Autodesk Inventor part; units mm, degrees
ref_plane "YZ Plane" through (0, 0, 0) normal (1, 0, 0) x (0, 1, 0)
ref_plane "XZ Plane" through (0, 0, 0) normal (0, 1, 0) x (-1, 0, 0)
ref_plane "XY Plane" through (0, 0, 0) normal (0, 0, 1) x (1, 0, 0)
sketch "Skizze1" plane through (0, 0, 0) normal (0, 0, 1) x (1, 0, 0)
  line L0 (-80, 62.5) -> (80, 62.5)
  line L1 (80, 62.5) -> (80, -62.5)
  line L2 (80, -62.5) -> (-80, -62.5)
  line L3 (-80, -62.5) -> (-80, 62.5)
  line L4 (-80, 62.5) -> (80, -62.5) construction
  line L5 (80, 62.5) -> (-80, -62.5) construction
  point P0 (0, 0)
  dimension "d0" = 160
  dimension "d1" = 125
extrude "Extrusion1" add sketch "Skizze1" along normal blind 5
fillet "Rundung1" radius 20 4 edges at (80, 62.5, 2.5) (80, -62.5, 2.5) (-80, -62.5, 2.5) (-80, 62.5, 2.5)
sketch "Skizze2" plane through (0, 0, 5) normal (0, 0, 1) x (1, 0, 0)
  line L0 (6.6667, 14.6667) -> (14.6667, 14.6667)
  line L1 (14.6667, 14.6667) -> (14.6667, 6.6667)
  line L2 (14.6667, 6.6667) -> (6.6667, 6.6667)
  line L3 (6.6667, 6.6667) -> (6.6667, 14.6667)
  line L4 (6.6667, 14.6667) -> (14.6667, 6.6667) construction
  line L5 (14.6667, 14.6667) -> (6.6667, 6.6667) construction
  line L6 (2.6667, 18.6667) -> (18.6667, 18.6667)
  line L7 (18.6667, 18.6667) -> (18.6667, 2.6667)
  line L8 (18.6667, 2.6667) -> (2.6667, 2.6667)
  line L9 (2.6667, 2.6667) -> (2.6667, 18.6667)
  line L10 (2.6667, 18.6667) -> (18.6667, 2.6667) construction
  line L11 (18.6667, 18.6667) -> (2.6667, 2.6667) construction
  line L12 (-1.3333, 22.6667) -> (22.6667, 22.6667)
  line L13 (22.6667, 22.6667) -> (22.6667, -1.3333)
  line L14 (22.6667, -1.3333) -> (-1.3333, -1.3333)
  line L15 (-1.3333, -1.3333) -> (-1.3333, 22.6667)
  line L16 (-1.3333, 22.6667) -> (22.6667, -1.3333) construction
  line L17 (22.6667, 22.6667) -> (-1.3333, -1.3333) construction
  line L18 (-10.6667, -10.6667) -> (10.6667, -10.6667) construction
  line L19 (10.6667, -10.6667) -> (10.6667, 10.6667) construction
  line L20 (10.6667, 10.6667) -> (-10.6667, 10.6667) construction
  line L21 (-10.6667, 10.6667) -> (-10.6667, -10.6667) construction
  line L22 (-10.6667, -10.6667) -> (10.6667, 10.6667) construction
  line L23 (10.6667, -10.6667) -> (-10.6667, 10.6667) construction
  line L24 (60, 62.5) -> (-60, 62.5) construction
  line L25 (80, -42.5) -> (80, 42.5) construction
  line L26 (-14.6667, -14.6667) -> (-14.6667, -6.6667)
  line L27 (-14.6667, -6.6667) -> (-6.6667, -6.6667)
  line L28 (-6.6667, -6.6667) -> (-6.6667, -14.6667)
  line L29 (-6.6667, -14.6667) -> (-14.6667, -14.6667)
  line L30 (-6.6667, -6.6667) -> (-14.6667, -14.6667) construction
  line L31 (-2.6667, -2.6667) -> (-2.6667, -18.6667)
  line L32 (-18.6667, -2.6667) -> (-2.6667, -2.6667)
  line L33 (-18.6667, -18.6667) -> (-18.6667, -2.6667)
  line L34 (-2.6667, -18.6667) -> (-18.6667, -18.6667)
  line L35 (-2.6667, -2.6667) -> (-18.6667, -18.6667) construction
  line L36 (-18.6667, -2.6667) -> (-2.6667, -18.6667) construction
  line L37 (1.3333, -22.6667) -> (-22.6667, -22.6667)
  line L38 (-22.6667, 1.3333) -> (1.3333, 1.3333)
  line L39 (-22.6667, -22.6667) -> (-22.6667, 1.3333)
  line L40 (1.3333, 1.3333) -> (1.3333, -22.6667)
  line L41 (-22.6667, 1.3333) -> (1.3333, -22.6667) construction
  line L42 (1.3333, 1.3333) -> (-22.6667, -22.6667) construction
  line L43 (-14.6667, -6.6667) -> (-6.6667, -14.6667) construction
  point P0 (0, 0)
  point P1 (1.3333, -1.3333)
  point P2 (-1.3333, 1.3333)
  dimension "d14" = 8
  dimension "d15" = 8
  dimension "d16" = 16
  dimension "d17" = 16
  dimension "d18" = 24
  dimension "d20" = 21.3333
  dimension "d21" = 21.3333
  dimension "d22" = 62.5
  dimension "d23" = 80
  dimension "d24" = 8
  dimension "d25" = 8
  dimension "d26" = 16
  dimension "d27" = 16
  dimension "d28" = 24
extrude "Extrusion2" cut sketch "Skizze2" against normal blind 1.5
sketch "Skizze3" plane through (0, 0, 0) normal (0, 0, -1) x (-1, 0, 0)
  circle A0 centre (50, -53.5) radius 4
  line L0 (60, -62.5) -> (-60, -62.5)
  line L1 (80, 42.5) -> (80, -42.5)
  line L2 (50, -53.5) -> (-45.5, -53.5)
  line L3 (-45.5, -53.5) -> (-45.5, 25)
  line L4 (-45.5, 25) -> (50, 25)
  line L5 (50, 25) -> (50, -53.5)
  circle A1 centre (-45.5, -53.5) radius 4
  circle A2 centre (-45.5, 25) radius 4
  circle A3 centre (50, 25) radius 4
  circle A4 centre (-45.5, 25) radius 2
  circle A5 centre (50, 25) radius 2
  circle A6 centre (50, -53.5) radius 2
  circle A7 centre (-45.5, -53.5) radius 2
  point P0 (0, 0)
  dimension "d31" = 9
  dimension "d32" = 30
  dimension "d33" = 8
  dimension "d34" = 78.5
  dimension "d35" = 95.5
  dimension "d36" = 8
  dimension "d37" = 8
  dimension "d38" = 8
  dimension "d39" = 4
  dimension "d40" = 4
  dimension "d41" = 4
  dimension "d42" = 4
extrude "Extrusion3" add sketch "Skizze3" along normal blind 7 contours A0 L2 A6 L5 | L5 A6 L2 A0 | A3 L4 A5 L5 | L5 A5 L4 A3 | A1 L3 A7 L2 | L2 A7 L3 A1 | A2 L3 A4 L4 | L4 A4 L3 A2
sketch "Skizze4" plane through (0, 0, 0) normal (0, 0, -1) x (-1, 0, 0)
  line L0 (-80, -42.5) -> (-80, 42.5)
  line L1 (80, 42.5) -> (80, -42.5)
  line L2 (-77, 40) -> (-65, 40)
  line L3 (-65, 40) -> (-65, -40)
  line L4 (-65, -40) -> (-77, -40)
  line L5 (-77, -40) -> (-77, 40)
  line L6 (77, 40) -> (65, 40)
  line L7 (65, 40) -> (65, -40)
  line L8 (65, -40) -> (77, -40)
  line L9 (77, -40) -> (77, 40)
  point P0 (0, 0)
  point P1 (-71, 40)
  dimension "d45" = 3
  dimension "d46" = 80
  dimension "d47" = 40
  dimension "d48" = 12
  dimension "d49" = 3
  dimension "d50" = 12
  dimension "d51" = 80
  dimension "d52" = 40
extrude "Extrusion4" add sketch "Skizze4" along normal blind 25
sketch "Skizze5" plane through (77, -40, 0) normal (1, 0, 0) x (0, 0, -1)
  line L0 (0, 0) -> (0, 80)
  line L1 (0, 0) -> (25, 0)
  line L2 (25, 80) -> (25, 0)
  line L3 (0, 80) -> (25, 80)
  line L4 (0, -2.5) -> (0, 82.5)
  point P0 (0, 40)
  point P1 (15, 70)
  point P2 (15, 10)
  point P3 (0, 40)
  point P4 (0, 40)
  dimension "d55" = 30
  dimension "d56" = 30
  dimension "d57" = 15
  dimension "d58" = 15
hole "Bohrung1" at (77, 30, -15) at (77, -30, -15) direction (-1, 0, 0) diameter 5.6 depth 154
chamfer "Fasen1" distance 2 angle 45 2 edges at (77, 0, -25) (-77, 0, -25)
equation "\"d14\" = d24"
equation "\"d15\" = d14"
equation "\"d16\" = 2 * d14"
equation "\"d17\" = d16"
equation "\"d18\" = 3 * d14"
equation "\"d20\" = 2.66667 * d24"
equation "\"d21\" = d20"
equation "\"d25\" = d24"
equation "\"d26\" = 2 * d24"
equation "\"d27\" = d26"
equation "\"d28\" = 3 * d24"
properties part number "240_Backplate"
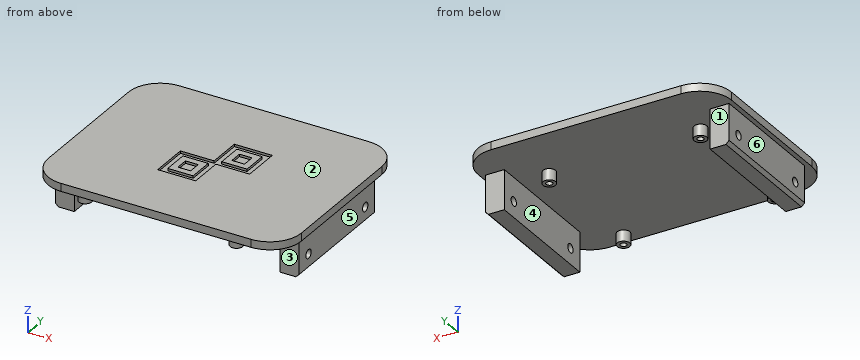
Here's how the part is built. I have some questions about the finished solid (model axes, mm). Face numbers are marked on the shaded views. A direction names the side the tool comes from. Give positions to 0.01 mm unless a question says otherwise; leave off trailing zeros. Order: outer loops, then holes, each group sorted by start corner. A loop starts at its lowest first (then second) coordinate and runs counter-clockwise, first axis right, second up. Notation, with made-up numbers: (43, 9.5) - (74, 9.5) arc R23 ccw to (74, 22.5) - close; hole circle Ø5 at (-11, -24.75). An arc over 180 degrees is marked (long way). Answer as a JSON object with one key per item and string values. Group by question number.
Item 1: If we section it at A-A on z = -2.25: Give the number of separate pieces and of enclosed holes in the cut face, and give its area (3 significant figures).
Item 2: If we mould it in two halves opening along X, with no side actions, what happens to the marked faces 4, 5 and 6? For each: pulls with the +X half, pulls with the -X half, needs draft (parallel to the pull), parting line crosses it, or undercut.
Item 3: Please list where these lines run through material, in increasing order: probe 1 along Y at (x, z) = (-50, -1.25); probe 2 along X at (y, z) = (-53.5, -4.5); probe 3 along Y at (x, z) = (74, -15).
Item 4: Which directions (+Z, -Z, +X, -X, +Y, -Y) give clear straight access to the entire face, cutting with the end or side of a thin tool? Please do the marked faces 1, 2 and 3.
Item 5: If we section it at D-D on x = 45.5: Please give me the cut outline in (y, z).
Item 6: If we section it at C-C on z = -20.5: Please give me the cut outline in (x, y).
Item 7: If we section it at B-B on y = -30: Please give me the cut outline in (x, z).
Item 8: For P1, Ø4, axis at y = -5.5, z = -12.5, coming from the -X side; P2, Ø9.5, axis at x = 72.5, z = -17.5, coming from the -Y side; P3, Ø4.5, axis at x = -50, y = -53.5, coming from the -Z side; P4, Ø4, axis at x = 17, z = -3.5, coming from the +Y side, each with a flat end and sliding along its axis, tell me the tip position at first contact or that it passes through.
Result set:
{
 "1": {"separate pieces": "6", "enclosed holes": "4", "area": "2,070 mm²"},
 "2": {"face 4": "undercut", "face 5": "pulls with the +X half", "face 6": "pulls with the -X half"},
 "3": {"probe 1": "-57.5 to -55.5, -51.5 to -49.5, 21 to 23, 27 to 29", "probe 2": "-54 to -52, -48 to -46, 41.5 to 43.5, 47.5 to 49.5", "probe 3": "-40 to -32.8, -27.2 to 27.2, 32.8 to 40"},
 "4": {"face 1": "-Z, +X, -X, +Y", "face 2": "+Z, +X, -X, +Y, -Y", "face 3": "-Z, +X, -X, -Y"},
 "5": {"outline": "(-62.5, 0) - (-57.5, 0) - (-57.5, -7) - (-55.5, -7) - (-55.5, 0) - (-51.5, 0) - (-51.5, -7) - (-49.5, -7) - (-49.5, 0) - (21, 0) - (21, -7) - (23, -7) - (23, 0) - (27, 0) - (27, -7) - (29, -7) - (29, 0) - (62.5, 0) - (62.5, 5) - (-62.5, 5) - close"},
 "6": {"outline": "(-77, -40) - (-65, -40) - (-65, 40) - (-77, 40) - close; (65, -40) - (77, -40) - (77, 40) - (65, 40) - close"},
 "7": {"outline": "(-80, 0) - (-77, 0) - (-77, -12.2) - (-65, -12.2) - (-65, 0) - (65, 0) - (65, -12.2) - (77, -12.2) - (77, 0) - (80, 0) - (80, 5) - (-80, 5) - close; (-77, -23) - (-75, -25) - (-65, -25) - (-65, -17.8) - (-77, -17.8) - close; (65, -25) - (75, -25) - (77, -23) - (77, -17.8) - (65, -17.8) - close"},
 "8": {"P1": "x = -77", "P2": "y = -40", "P3": "z = -7", "P4": "through"}
}
